Source: CAD feature listing. Evaluate the final solid. Frame: model axes, mm. Face numbers are marked on the shaded views. Round coordinates to 2 decimals unless told otherwise and drop trailing zeros. Order: outer loops, then holes, each group sorted by start corner. A loop starts at its lowest first (then second) coordinate and runs counter-clockwise, first axis right, second up. Notation, with made-up numbers: (12.5, 40.25) -> (34.5, 40.25) arc R13 cw to (34.5, 50.25) -> close; hole circle Ø3 at (38.25, -21). An arc over 180 degrees is marked (long way). One line per item, written item: value. Start each with the question number.
1) Mould query, pull axis Z, two halves, no side actions, for the marked faces 1, 2 and 3. Classes: pulls with the +Z half, pulls with the -Z half, needs draft (parallel to the pull), parting line crosses it, or undercut.
2) Pin query (flat end, axial travel): P1, Ø1.5, axis at x = 7.5, y = -2, coming from the +Z side; P2, Ø1, axis at y = -1, z = 15, coming from the +X side; P3, Ø3, axis at x = -5, y = -4.5, coming from the +Z side. Return the tip coordinate at first contact, or that it passes through.
3) Section C-C (z = -13). Return the cut outline in (x, y), and give its area (3 significant figures).
4) Ray query, L1, parallel to Z at x = 0, y = -1.15; L2, parallel to X at y = -2.5, z = -3.7; L3, parallel to Z at x = 11, y = -2.65. Return the intervals inside material, ascending.
5) Section B-B (x = 9). Return the cut outline in (y, z), and give its area (3 significant figures).
6) Section A-A (y = -2.5). State how many separate pieces and enclosed holes the cut face has, and give its area (3 significant figures).
7) Section D-D (y = -4.4). Return the cut outline in (x, z), and give its area (3 significant figures).
```python
from build123d import *

# Parameters (mm, degrees)
F0_R     = 2.5
F1_DEPTH = 5
F2_R     = 5
F3_R     = 1.5
F4_DEPTH = 25
F5_R     = 1


with BuildPart() as f1:
    # F0 (on Front) → F1 (new body)
    with BuildSketch(Plane.XZ):
        with BuildLine():
            ThreePointArc((3.968627, -0.5), (-4, 0), (3.968627, 0.5))
            Line((3.968627, 0.5), (12.5, 0.5))
            Line((12.5, 0.5), (12.5, 5))
            Line((12.5, 5), (6, 5))
            Line((6, 5), (4.976343, 15.485806))
            ThreePointArc((4.976343, 15.485806), (0.813163, 19.933434), (-4.557189, 17.057189))
            Line((-4.557189, 17.057189), (-10, 5))
            Line((-10, 5), (-10, -5))
            Line((-10, -5), (-4.557189, -17.057189))
            ThreePointArc((-4.557189, -17.057189), (0.813163, -19.933434), (4.976343, -15.485806))
            Line((4.976343, -15.485806), (6, -5))
            Line((6, -5), (12.5, -5))
            Line((12.5, -5), (12.5, -0.5))
            Line((12.5, -0.5), (3.968627, -0.5))
        make_face()
        with Locations((0, -15)):
            Circle(F0_R, mode=Mode.SUBTRACT)
        with Locations((0, 15)):
            Circle(F0_R, mode=Mode.SUBTRACT)
    extrude(amount=F1_DEPTH)

    # F2
    f2_edges = [f1.edges().sort_by_distance(p)[0] for p in [
        (-10, -2.5, -5),
        (-10, -2.5, 5),
    ]]
    fillet(f2_edges, radius=F2_R)

    # F3 (on face) → F4 (cut)
    with BuildSketch(Plane(origin=(0, 0, -5), x_dir=(1, 0, 0), z_dir=(0, 0, -1))):
        with Locations((9, 2.5)):
            Circle(F3_R)
    extrude(amount=-F4_DEPTH, mode=Mode.SUBTRACT)

    # F5
    f5_edges = [f1.edges().sort_by_distance(p)[0] for p in [
        (6, -2.5, -5),
        (12.5, -2.5, -5),
        (12.5, -2.5, 5),
        (6, -2.5, 5),
        (12.5, -2.5, 0.5),
        (12.5, -2.5, -0.5),
        (3.968627, -2.5, -0.5),
        (3.968627, -2.5, 0.5),
    ]]
    fillet(f5_edges, radius=F5_R)


solid = f1.part
```
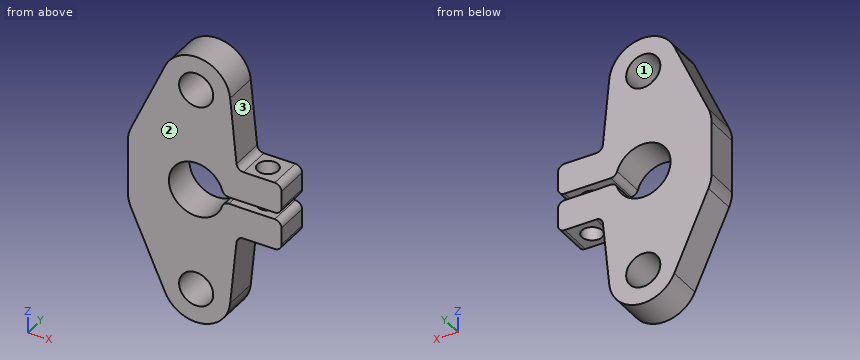
Findings:
1. face 1: undercut
1. face 2: needs draft
1. face 3: pulls with the +Z half
2. P1: z = 5.01
2. P2: x = 5.07
2. P3: z = 18.57
3. outline: (-6.39, -5) -> (-1.5, -5) -> (-1.5, 0) -> (-6.39, 0) -> close; (1.5, -5) -> (5.22, -5) -> (5.22, 0) -> (1.5, 0) -> close
3. area: 43.0 mm2
4. L1: -20 to -17.5, -12.5 to -4, 4 to 12.5, 17.5 to 20
4. L2: -10 to -1.52, 1.52 to 7.5, 10.5 to 12.5
4. L3: -5 to -0.5, 0.5 to 5
5. outline: (-5, -5) -> (-4, -5) -> (-4, -0.5) -> (-5, -0.5) -> close; (-5, 0.5) -> (-4, 0.5) -> (-4, 5) -> (-5, 5) -> close; (-1, -5) -> (0, -5) -> (0, -0.5) -> (-1, -0.5) -> close; (-1, 0.5) -> (0, 0.5) -> (0, 5) -> (-1, 5) -> close
5. area: 18.0 mm2
6. separate pieces: 3
6. enclosed holes: 2
6. area: 443 mm2
7. outline: (-10, -3.92) arc R5 ccw to (-9.56, -5.98) -> (-4.56, -17.06) arc R5 ccw to (4.98, -15.49) -> (5.91, -5.9) arc R1 cw to (6.91, -5) -> (11.5, -5) arc R1 ccw to (12.5, -4) -> (12.5, -1.5) arc R1 ccw to (11.5, -0.5) -> (4.77, -0.5) arc R1 ccw to (3.82, -1.2) arc R4 cw (long way) to (3.82, 1.2) arc R1 ccw to (4.77, 0.5) -> (11.5, 0.5) arc R1 ccw to (12.5, 1.5) -> (12.5, 4) arc R1 ccw to (11.5, 5) -> (6.91, 5) arc R1 cw to (5.91, 5.9) -> (4.98, 15.49) arc R5 ccw to (-4.56, 17.06) -> (-9.56, 5.98) arc R5 ccw to (-10, 3.92) -> close; hole circle Ø5 at (0, -15); hole circle Ø5 at (0, 15)
7. area: 470 mm2
